```python
from build123d import *

# Parameters (mm, degrees)
EXTRUDE_THIN1_DEPTH      = 240
EXTRUDE_THIN1_DEPTH_BACK = 240
CUT_EXTRUDE1_REACH       = 242.754
LPATTERN1_COUNT          = 10
LPATTERN1_PITCH          = 25
LPATTERN1_COL_COUNT      = 10
LPATTERN1_COL_PITCH      = 25


with BuildPart() as part:
    # Sketch1 → Extrude-Thin1 (new, two sides: drawn at the far end of the back side and taken through both)
    with BuildSketch(Plane(origin=(0, 0, 0), x_dir=(0, 0, -1), z_dir=(1, 0, 0)).offset(-EXTRUDE_THIN1_DEPTH_BACK)):
        with BuildLine():
            Line((-17.5, 6.5), (-15.5, 6.5))
            ThreePointArc((-15.5, 6.5), (-14.085786438, 5.914213562), (-13.5, 4.5))
            Line((-13.5, 4.5), (-13.5, 2))
            ThreePointArc((-13.5, 2), (-12.914213562, 0.585786438), (-11.5, 0))
            Line((-11.5, 0), (11.5, 0))
            ThreePointArc((11.5, 0), (12.914213562, 0.585786438), (13.5, 2))
            Line((13.5, 2), (13.5, 4.5))
            ThreePointArc((13.5, 4.5), (14.085786438, 5.914213562), (15.5, 6.5))
            Line((15.5, 6.5), (17.5, 6.5))
            Line((17.5, 6.5), (17.5, 7.5))
            Line((17.5, 7.5), (15.5, 7.5))
            ThreePointArc((15.5, 7.5), (13.378679656, 6.621320344), (12.5, 4.5))
            Line((12.5, 4.5), (12.5, 2))
            ThreePointArc((12.5, 2), (12.207106781, 1.292893219), (11.5, 1))
            Line((11.5, 1), (-11.5, 1))
            ThreePointArc((-11.5, 1), (-12.207106781, 1.292893219), (-12.5, 2))
            Line((-12.5, 2), (-12.5, 4.5))
            ThreePointArc((-12.5, 4.5), (-13.378679656, 6.621320344), (-15.5, 7.5))
            Line((-15.5, 7.5), (-17.5, 7.5))
            Line((-17.5, 7.5), (-17.5, 6.5))
        make_face()
    extrude(amount=EXTRUDE_THIN1_DEPTH + EXTRUDE_THIN1_DEPTH_BACK)

    # Sketch2 → Cut-Extrude1 (cut, up to next)
    with BuildSketch(Plane.XZ, mode=Mode.PRIVATE) as cut_extrude1_sk1:
        with BuildLine():
            Line((-5.875, 3.125), (5.875, 3.125))
            ThreePointArc((5.875, 3.125), (9, 0), (5.875, -3.125))
            Line((5.875, -3.125), (-5.875, -3.125))
            ThreePointArc((-5.875, -3.125), (-9, 0), (-5.875, 3.125))
        make_face()
    cut_extrude1_tool1 = extrude(cut_extrude1_sk1.sketch, amount=-CUT_EXTRUDE1_REACH, mode=Mode.PRIVATE) & part.part
    cut_extrude1 = cut_extrude1_tool1.solids().sort_by_distance((0, 0, 0))[0]
    add(cut_extrude1, mode=Mode.SUBTRACT)

    # LPattern1: Cut-Extrude1 ×10
    with Locations(*[(i * LPATTERN1_PITCH, 0, 0) for i in range(1, LPATTERN1_COUNT)]):
        add(cut_extrude1, mode=Mode.SUBTRACT)

    # LPattern1 col: Cut-Extrude1 ×10
    with Locations(*[(-i * LPATTERN1_COL_PITCH, 0, 0) for i in range(1, LPATTERN1_COL_COUNT)]):
        add(cut_extrude1, mode=Mode.SUBTRACT)


solid = part.part
```
Work out the finished part from the listing and answer in its coordinate system (mm). Coordinates: 2 decimals unless noted, no trailing zeros. Write each loop counter-clockwise with the first axis right and the second up, starting at its lowest first coordinate (ties: lowest second). Pieces come first, ordered by that corner, then holes.
Q1. Determine the mould class of faces 1 (the face through (-3, 0, 5)), 2 (the face through (-3, 1, -5)) for opening direction Z: released by +Z, released by -Z, zero draft, split by the parting line, or undercut.
Q2. Find the intervals of material crossed by line 1 (Z direction, x = -163, y = 4.25); line 2 (Z direction, x = 22, y = 6); line 3 (Y direction, x = 35, z = -9), in increasing order.
Q3. A cutting plane is placed at A-A, the plane z = -7.5. Give the vertices of the cut face in (x, y).
Q4. Each of these flat-tipped pins is pushed along its axis until it touches: pin 1 Ø0.8 at (x, y) = (-174.5, 0.5) entering from -Z; pin 2 Ø2 at (x, z) = (10, 11) entering from +Y; pin 3 Ø3 at (x, y) = (57, 2) entering from +Z. Where does it stop, or does it pass through?
Findings below:
1. face 1: zero draft
1. face 2: undercut
2. line 1: z = -13.5 to -12.5, 12.5 to 13.5
2. line 2: z = -14.18 to -12.9, 12.9 to 14.18
2. line 3: y = 0 to 1
3. outline: (-240, 0) - (240, 0) - (240, 1) - (-240, 1) - close
4. pin 1: stops at z = -13.17
4. pin 2: stops at y = 1.13
4. pin 3: stops at z = 13.5
